Read the model definition and answer for the solid it produces. Units are mm, in the model's axes. Coordinates: 2 decimals unless noted, no trailing zeros. Order: outer loops, then holes, each group sorted by start corner. A loop starts at its lowest first (then second) coordinate and runs counter-clockwise, first axis right, second up.
```python
from build123d import *

# Parameters (mm, degrees)
SKETCH1_R               = 14
SKETCH1_R_2             = 12.4125
BOSS_EXTRUDE1_DEPTH     = 650
SKETCH2_R               = 2.5
CUT_EXTRUDE2_DEPTH      = 15
CUT_EXTRUDE2_DEPTH_BACK = 15
SKETCH6_R               = 2.5
CUT_EXTRUDE4_DEPTH      = 15.0000001
CUT_EXTRUDE4_DEPTH_BACK = 15.0000001


with BuildPart() as part:
    # Sketch1 → Boss-Extrude1 (new body)
    with BuildSketch(Plane(origin=(0, 0, 0), x_dir=(1, 0, 0), z_dir=(0, 1, 0))):
        Circle(SKETCH1_R)
        Circle(SKETCH1_R_2, mode=Mode.SUBTRACT)
    extrude(amount=BOSS_EXTRUDE1_DEPTH)

    # Sketch2 → Cut-Extrude2 (cut, two sides)
    with BuildSketch(Plane.XY) as cut_extrude2_sk:
        with Locations((0, 10)):
            Circle(SKETCH2_R)
        with Locations((0, 640)):
            Circle(SKETCH2_R)
    extrude(amount=CUT_EXTRUDE2_DEPTH, mode=Mode.SUBTRACT)
    extrude(cut_extrude2_sk.sketch, amount=-CUT_EXTRUDE2_DEPTH_BACK, mode=Mode.SUBTRACT)

    # Sketch6 → Cut-Extrude4 (cut, two sides)
    with BuildSketch(Plane(origin=(0, 0, 0), x_dir=(0, 0, -1), z_dir=(1, 0, 0))) as cut_extrude4_sk:
        with Locations((0, 285)):
            Circle(SKETCH6_R)
        with Locations((0, 275)):
            Circle(SKETCH6_R)
    extrude(amount=CUT_EXTRUDE4_DEPTH, mode=Mode.SUBTRACT)
    extrude(cut_extrude4_sk.sketch, amount=-CUT_EXTRUDE4_DEPTH_BACK, mode=Mode.SUBTRACT)


solid = part.part
```
1) Straight lines are drawn through the part: line 1 (Y direction, x = 0, z = 13.5); line 2 (Z direction, x = -0.25, y = 133). For each, find the intervals that lie inside material, in ascending order.
A:
line 1: y = 0 to 7.5, 12.5 to 637.5, 642.5 to 650
line 2: z = -14 to -12.41, 12.41 to 14
2) Determine the mould class of faces 1 (the flat face through (-2.1, 650, 12.4)), 2 (the cylindrical face through (-9.85, 320.45, 7.55)), 3 (the cylindrical face through (12.932, 320.45, 5.362)) for opening direction Z: pulls with the +Z half, pulls with the -Z half, needs draft (parallel to the pull), parting line crosses it, or undercut.
A:
face 1: needs draft
face 2: undercut
face 3: parting line crosses it
3) A cutting plane is placed at B-B, the plane y = 404. Determine the outline of the cut face in (x, z) (1 decimal).
A:
outline: circle Ø28 at (0, 0); hole circle Ø24.8 at (0, 0)
4) A cutting plane is placed at C-C, the plane z = -6.75. Determine the outline of the cut face in (x, y).
A:
outline: (-12.27, 0) - (-10.42, 0) - (-10.42, 650) - (-12.27, 650) - close; (10.42, 0) - (12.27, 0) - (12.27, 650) - (10.42, 650) - close
5) A cutting plane is placed at A-A, the plane x = 7. Determine the outline of the cut face in (y, z), and give its area (3 significant figures).
A:
outline: (0, -12.12) - (650, -12.12) - (650, -10.25) - (0, -10.25) - close; (0, 10.25) - (650, 10.25) - (650, 12.12) - (0, 12.12) - close
area: 2,440 mm2
6) Flat-ended cylindrical pins translate along their axes: pin 1 Ø1 at (x, y) = (10, 533) entering from +Z; pin 2 Ø4.5 at (x, y) = (0, 640) entering from -Z; pin 3 Ø1 at (y, z) = (430, 8.5) entering from -X; pin 4 Ø1.5 at (x, y) = (-4.5, 370) entering from -Z. Find the tip coordinate at first contact, or state that the pin passes through.
A:
pin 1: stops at z = 10.28
pin 2: passes through
pin 3: stops at x = -11.49
pin 4: stops at z = -13.49
